Work out the finished part from the listing and answer in its coordinate system (mm). A direction names the side the tool comes from. Round coordinates to 2 decimals unless told otherwise and drop trailing zeros. Loops run counter-clockwise (first coordinate to the right, second up) from the corner with the lowest first, then second, coordinate; pieces in that order, holes last. Notation, with made-up numbers: (-4.5, -24.75) - (35.5, -24.75) arc R31 ccw to (35.5, 6.25) - close; hole circle Ø1 at (18.25, 84.5). An arc over 180 degrees is marked (long way). Use CSV: the item, a comma, the result in double quotes. Start each with the question number.
from build123d import *

# Parameters (mm, degrees)
SKETCH025_R              = 8
PAD014_DEPTH             = 8
SKETCH026_R              = 6
PAD015_DEPTH             = 7.25
SKETCH027_R              = 0.5
POCKET008_DEPTH          = 7.25
POLARPATTERN_COUNT       = 20
SKETCH028_R              = 8
PAD016_DEPTH             = 1.25
SKETCH029_R              = 2.5
POCKET009_DEPTH          = 16.5
CLONE005_PLACEMENT_ANGLE = 180


with BuildPart() as part:
    # Sketch025 → Pad014 (new body)
    with BuildSketch(Plane(origin=(20, -80, 0), x_dir=(1, 0, 0), z_dir=(0, 0, -1))):
        Circle(SKETCH025_R)
    extrude(amount=PAD014_DEPTH)

    # Sketch026 → Pad015 (new body)
    with BuildSketch(Plane(origin=(20, -80, -8), x_dir=(1, 0, 0), z_dir=(0, 0, -1))):
        Circle(SKETCH026_R)
    extrude(amount=PAD015_DEPTH)

    # Sketch027 → Pocket008 (cut)
    with BuildSketch(Plane(origin=(20, -80, -15.25), x_dir=(1, 0, 0), z_dir=(0, 0, -1))):
        with Locations((6, 0)):
            Circle(SKETCH027_R)
    pocket008 = extrude(amount=-POCKET008_DEPTH, mode=Mode.SUBTRACT)

    # PolarPattern: Pocket008 ×20 about axis
    polarpattern_axis = Axis((20, -80, -15.25), (0, 0, -1))
    for i in range(1, POLARPATTERN_COUNT):
        add(pocket008.rotate(polarpattern_axis, i * 360 / POLARPATTERN_COUNT), mode=Mode.SUBTRACT)

    # Sketch028 → Pad016 (new body)
    with BuildSketch(Plane(origin=(20, -80, -15.25), x_dir=(1, 0, 0), z_dir=(0, 0, -1))):
        Circle(SKETCH028_R)
    extrude(amount=PAD016_DEPTH)

    # Sketch029 → Pocket009 (cut)
    with BuildSketch(Plane(origin=(20, -80, -16.5), x_dir=(1, 0, 0), z_dir=(0, 0, -1))):
        Circle(SKETCH029_R)
    extrude(amount=-POCKET009_DEPTH, mode=Mode.SUBTRACT)


with BuildPart() as part_1:
    # Clone005 placement: moved
    add(part.part.moved(Location((-6, -192, -13))).rotate(Axis((-6, -192, -13), (-1, 0, 0)), CLONE005_PLACEMENT_ANGLE))


solid = part_1.part
Item 1: Find the intervals of material crossed by probe 1 along Y at (x, z) = (14, 0); probe 2 along Z at (x, y) = (15.5, -105.75); probe 3 along X at (y, z) = (-108.5, -3.5), in increasing order. Write a range as [from, to].
Item 2: The mould has two halves that part along X. Classify faces 4 (the cylindrical face through (12.27, -119.81, -9.06)), 5 (the cylindrical face through (14.932, -117.927, -1.426)), 6 (the cylindrical face through (12.311, -117.234, -1.324)): pulls with the +X half, pulls with the -X half, needs draft (parallel to the pull), parting line crosses it, or undercut.
Item 3: A cutting plane is placed at D-D (y = -108.5). Determine the outline of the cut face in (x, z).
Item 4: A cutting plane is placed at B-B (y = -105.5). Determine the outline of the cut face in (x, z).
Item 5: Each of these flat-tipped pins is pushed along its axis until it touches: pin 1 Ø3 at (x, z) = (12.5, 0) entering from +Y; pin 2 Ø5 at (y, z) = (-116, -6) entering from -X; pin 3 Ø1 at (x, z) = (16.5, -11) entering from +Y. Where does it stop, or does it pass through?
Item 6: A cutting plane is placed at C-C (z = -6.5). Determine the outline of the cut face in (x, y).
Item 7: A cutting plane is placed at A-A (x = 14). Determine the outline of the cut face in (y, z), plus the area to 3 significant figures.
Item 8: Which of the six approach directions +Z, -Z, +X, -X, +Y, -Y give full straight-line access (tool end or side, diameter ignored) to faces 1 (the cylindrical face through (8.5, -112, -1.3)), 2 (the cylindrical face through (14.945, -106.075, -1.426)), 3 (the flat face through (8.6, -113.7, 2.25))?
Result sheet:
1,probe 1,"[-117.5, -114.5], [-109.5, -106.5]"
1,probe 2,"[-13, -5], [2.25, 3.5]"
1,probe 3,"[9.65, 18.35]"
2,face 4,"parting line crosses it"
2,face 5,"pulls with the +X half"
2,face 6,"undercut"
3,outline,"(6.81, -13) - (21.19, -13) - (21.19, -5) - (18.35, -5) - (18.35, 2.25) - (21.19, 2.25) - (21.19, 3.5) - (6.81, 3.5) - (6.81, 2.25) - (9.65, 2.25) - (9.65, -5) - (6.81, -5) - close"
4,outline,"(9.34, -13) - (18.66, -13) - (18.66, -5) - (9.34, -5) - close; (9.34, 2.25) - (18.66, 2.25) - (18.66, 3.5) - (9.34, 3.5) - close"
5,pin 1,"y = -106.02"
5,pin 2,"x = 6.14"
5,pin 3,"y = -104.25"
6,outline,"circle Ø16 at (14, -112); hole circle Ø5 at (14, -112)"
7,outline,"(-120, -13) - (-114.5, -13) - (-114.5, 3.5) - (-120, 3.5) - (-120, 2.25) - (-117.5, 2.25) - (-117.5, -5) - (-120, -5) - close; (-109.5, -13) - (-104, -13) - (-104, -5) - (-106.5, -5) - (-106.5, 2.25) - (-104, 2.25) - (-104, 3.5) - (-109.5, 3.5) - close"
7,area,"145 mm^2"
8,face 1,"-X"
8,face 2,"+X, +Y"
8,face 3,"none"
